Source: CAD feature listing. Evaluate the final solid. Frame: model axes, mm. A direction names the side the tool comes from. Give positions to 0.01 mm unless a question says otherwise; leave off trailing zeros. Write each loop counter-clockwise with the first axis right and the second up, starting at its lowest first coordinate (ties: lowest second). Pieces come first, ordered by that corner, then holes. Notation, with made-up numbers: (15.5, 21.5) -> (46.5, 21.5) arc R11 cw to (46.5, 30.5) -> close; hole circle Ø3 at (10, 0). An arc over 180 degrees is marked (long way). Answer as a JSON object with one key per item and string values. Group by question number.
Item 1: Section query C-C on z = 34. Return the cut outline in (x, y), plus the area to 3 significant figures.
Item 2: First-contact query: pin 1 Ø5 at (x, y) = (9.5, 14) entering from +Z; pin 2 Ø3.5 at (x, y) = (18, 24) entering from -Z; pin 3 Ø6 at (x, z) = (16.5, 16) entering from -Y. Flat tips, straight axial feed; report the tip coordinate or a pass-through.
Item 3: Access query for faces 1 (the face through (14.178, -3.226, 35.356)), 2 (the face through (13.03, 17.81, 1.6)), 3 (the face through (18.76, 4.39, 24.3)), 4 (the face through (17.49, 1.92, 30.87)), 5 (the face through (18.2, 0, 35)). Directions: +Z, -Z, +X, -X, +Y, -Y. A direction counts if a zero-diameter tool reaches every point of the face in a straight line with its end or side. Return the directions, or none.
Item 4: Section query A-A on y = 17. Return the cut outline in (x, z).
Item 5: Pull-direction query (Y, two-part tool) for faces 6 (the face through (15, 17.8, 18)), 7 (the face through (2, 2, 12)), 8 (the face through (20, 23, 21)); classes: pulls with the +Y half, pulls with the -Y half, needs draft (parallel to the pull), parting line crosses it, or undercut.
Item 6: Section query B-B on x = 8.5. Return the cut outline in (y, z).
Item 7: Ray query, probe 1 along Z at (x, y) = (2.25, 0.5); probe 2 along Y at (x, z) = (18.5, 9); probe 3 along X at (y, z) = (15, 16.5). Return the intervals inside material, ascending. Write a range as from..to.
Item 8: Section query D-D on y = 8. Return the cut outline in (x, z), plus the area to 3 significant figures.
from build123d import *

# Parameters (mm, degrees)
SKETCH_W             = 13.6
SKETCH_H             = 22.8
PAD_DEPTH            = 25.4
SKETCH001_W          = 3.2
SKETCH001_H          = 2
PAD001_DEPTH         = 17.8
PAD002_START         = -20.8
SKETCH002_W          = 20
SKETCH002_H          = 6
PAD002_DEPTH         = 4.6
SKETCH003_W          = 4.6
SKETCH003_H          = 13.6
POCKET_DEPTH         = 3.6
SKETCH005_W          = 19.6
SKETCH005_H          = 27.4
PAD003_DEPTH         = 10
PAD003_DEPTH_BACK    = 10
PAD004_DEPTH         = 19.6
SKETCH008_W          = 12.6
SKETCH008_H          = 3.6
SKETCH008_W_2        = 3.8
POCKET001_DEPTH      = 4.4
POCKET002_DEPTH      = 6.6
POCKET003_DEPTH      = 19.6
SKETCH011_W          = 4.6
SKETCH011_H          = 13.8
POCKET004_DEPTH      = 10
POCKET004_DEPTH_BACK = 2
FILLET_R             = 2.8
FILLET001_R          = 2


with BuildPart() as part:
    # Sketch → Pad (new body)
    with BuildSketch(Plane.XZ):
        with Locations((6.8, 12.4)):
            Rectangle(SKETCH_W, SKETCH_H)
    extrude(amount=-PAD_DEPTH)

    # Sketch001 → Pad001 (join)
    with BuildSketch(Plane.XZ):
        with Locations((15.2, 17.9)):
            Rectangle(SKETCH001_W, SKETCH001_H)
    extrude(amount=-PAD001_DEPTH)

    # Sketch002 → Pad002 (join)
    with BuildSketch(Plane.XZ.offset(PAD002_START)):
        with Locations((10, 20.8)):
            Rectangle(SKETCH002_W, SKETCH002_H)
    extrude(amount=-PAD002_DEPTH)

    # Sketch003 → Pocket (cut)
    with BuildSketch(Plane.XZ):
        with Locations((2.3, 11.4)):
            Rectangle(SKETCH003_W, SKETCH003_H)
    extrude(amount=-POCKET_DEPTH, mode=Mode.SUBTRACT)

    # Sketch005 → Pad003 (join, two sides)
    with BuildSketch(Plane.XZ) as pad003_sk:
        with Locations((9.8, 11.4)):
            Rectangle(SKETCH005_W, SKETCH005_H)
    extrude(amount=-PAD003_DEPTH)
    extrude(pad003_sk.sketch, amount=PAD003_DEPTH_BACK)

    # Sketch007 → Pad004 (join)
    with BuildSketch(Plane.YZ):
        Polygon((-1.2, 24.6), (-9.4692950629, 21.5902227387), (-14.3259810981, 34.9338579539), (-6.0566860352, 37.9436352152), (-4.8938175479, 34.7486803045), (-1.5109241131, 35.9799528205), (-2.2633684284, 38.0472765862), (0.5557094339, 39.0733370162), (3.6338907239, 30.6161034291), (0.8148128615, 29.5900429991), (-0.0060354825, 31.845305289), (-3.3889289173, 30.614032773), align=None)
    extrude(amount=PAD004_DEPTH)

    # Sketch008 (on DatumPlane) → Pocket001 (cut)
    with BuildSketch(Plane(origin=(0, -11.7404784812, 32.2566995207), x_dir=(-1, 0, 0), z_dir=(0, -0.3420201433, 0.9396926208))):
        with Locations((-6.3, -9.0860643809)):
            Rectangle(SKETCH008_W, SKETCH008_H)
        with Locations((-17.7, -9.0860643809)):
            Rectangle(SKETCH008_W_2, SKETCH008_H)
    extrude(amount=-POCKET001_DEPTH, mode=Mode.SUBTRACT)

    # Sketch009 (on DatumPlane) → Pocket002 (cut)
    with BuildSketch(Plane(origin=(0, 6.8466609333, 2.4919807838), x_dir=(1, 0, 0), z_dir=(0, 0.9396926208, 0.3420201433))):
        Polygon((11.600006173, -27.5268626433), (10.2, -29.195323), (10.2, -36.526867), (0, -36.526867), (0, -27.5268626433), align=None)
        Polygon((16.7999894706, -27.5268626433), (18.2, -29.1953225959), (18.2, -36.526867), (19.6, -36.526867), (19.6, -27.5268626433), align=None)
    extrude(amount=POCKET002_DEPTH, mode=Mode.SUBTRACT)

    # Sketch010 → Pocket003 (cut)
    with BuildSketch(Plane.YZ):
        Polygon((-0.773965096, -2.3), (-14.3259810981, -2.3), (-14.3259810981, 34.9338579539), align=None)
    extrude(amount=POCKET003_DEPTH, mode=Mode.SUBTRACT)

    # Sketch011 → Pocket004 (cut, two sides)
    with BuildSketch(Plane.XZ) as pocket004_sk:
        with Locations((2.3, 11.9)):
            Rectangle(SKETCH011_W, SKETCH011_H)
    extrude(amount=POCKET004_DEPTH, mode=Mode.SUBTRACT)
    extrude(pocket004_sk.sketch, amount=-POCKET004_DEPTH_BACK, mode=Mode.SUBTRACT)

    # Fillet
    fillet_edges = [part.edges().sort_by_distance(p)[0] for p in [
        (19.6, 4.309007, 25.1),
        (19.6, 4.613017, -2.3),
    ]]
    fillet(fillet_edges, radius=FILLET_R)

    # Fillet001
    fillet001_edges = [part.edges().sort_by_distance(p)[0] for p in [
        (13.6, 15.4, 23.8),
        (13.6, 17.7, 1),
    ]]
    fillet(fillet001_edges, radius=FILLET001_R)


solid = part.part
Worked answers:
{
 "1": {"outline": "(0, -13.99) -> (19.6, -13.99) -> (19.6, -4.62) -> (15.8, -4.62) -> (15.8, -0.79) -> (18.2, -0.79) -> (18.2, 2.4) -> (10.2, 2.4) -> (10.2, -0.79) -> (12.6, -0.79) -> (12.6, -4.62) -> (0, -4.62) -> close", "area": "221 mm^2"},
 "2": {"pin 1": "z = 23.8", "pin 2": "z = 17.8", "pin 3": "y = -8.53"},
 "3": {"face 1": "+X, -X", "face 2": "-Z, +X, +Y", "face 3": "+X", "face 4": "+X, +Y", "face 5": "+Z, +X, +Y"},
 "4": {"outline": "(0, 1) -> (11.6, 1) arc R2 ccw to (13.6, 3) -> (13.6, 16.9) -> (16.8, 16.9) -> (16.8, 18.9) -> (13.6, 18.9) -> (13.6, 21.8) arc R2 ccw to (11.6, 23.8) -> (0, 23.8) -> close"},
 "5": {"face 6": "undercut", "face 7": "pulls with the -Y half", "face 8": "needs draft"},
 "6": {"outline": "(-14.33, 34.93) -> (-0.77, -2.3) -> (10, -2.3) -> (10, 1) -> (25.4, 1) -> (25.4, 23.8) -> (10, 23.8) -> (10, 25.1) -> (-1.38, 25.1) -> (-6.06, 37.94) -> close"},
 "7": {"probe 1": "-2.3..5, 18.8..25.1", "probe 2": "-4.89..10", "probe 3": "0..13.6"},
 "8": {"outline": "(0, -2.3) -> (16.8, -2.3) arc R2.8 ccw to (19.6, 0.5) -> (19.6, 22.3) arc R2.8 ccw to (16.8, 25.1) -> (0, 25.1) -> close", "area": "534 mm^2"}
}
